The drawing under review shows one solid part. Ordinate dimensions are in mm from its lowest x, y, z. Give positions to 0.01 mm unless a question says otherwise; leave off trailing zeros. Loops run counter-clockwise (first coordinate to the right, second up) from the corner with the lowest first, then second, coordinate; pieces in that order, holes last. Notation, with made-up numbers: (46.5, 87) - (88.5, 87) arc R31 cw to (88.5, 117) - close; hole circle Ø11 at (6, 61). An arc over 180 degrees is marked (long way). One line per item, written item: value. Start each with the question number.
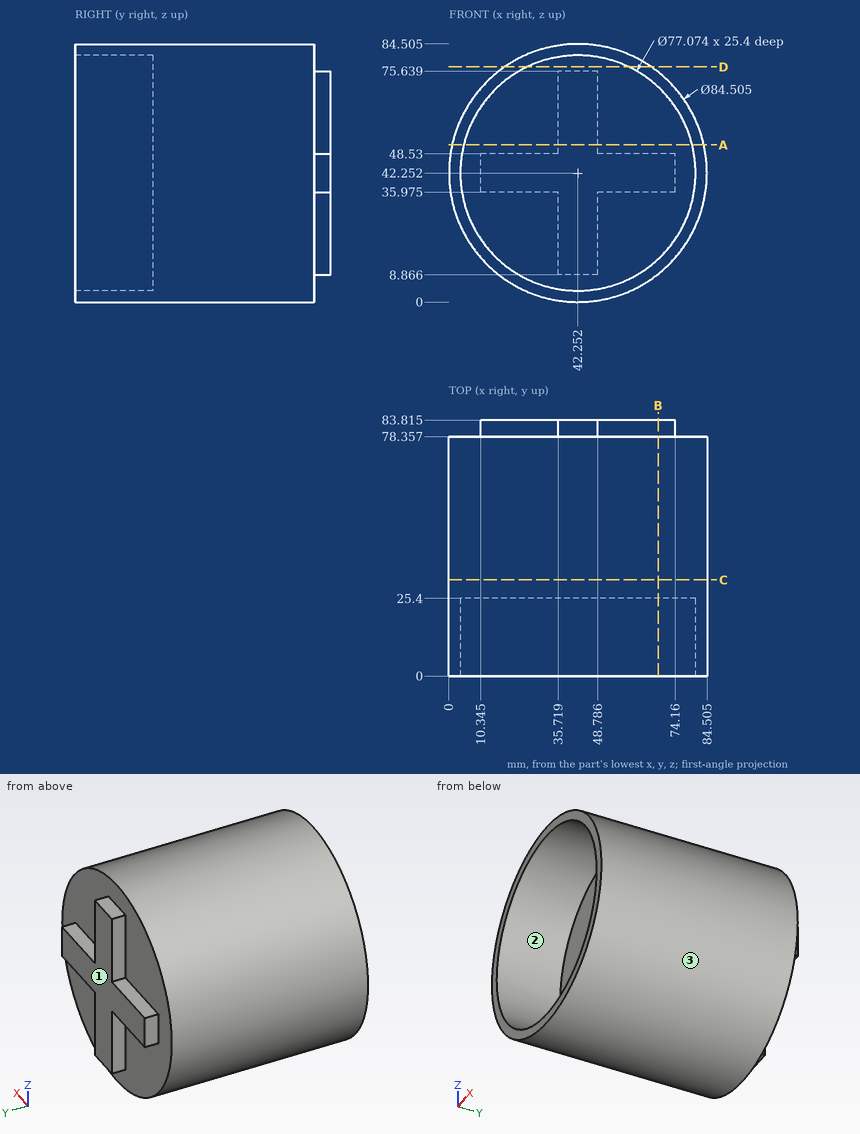
(1) To check wall thickness, follow L1, parallel to Y at x = 25, z = 58; L2, parallel to Y at x = 44, z = 17 (1 decimal); L3, parallel to X at y = 15, z = 13 (1 decimal). State the ranges of each line that lie inside material, in increasing order. Write a range as from..to.
(2) Take a section at B-B on x = 68.5. State the section outline as (y, z) points (1 decimal), and give its area (3 significant figures).
(3) Take a section at D-D on z = 77. State the section outline as (x, y) points, and give its area (3 significant figures).
(4) Take a section at A-A on z = 51.5. State the section outline as (x, y) points (1 decimal).
(5) Take a section at C-C on y = 31.5. State the section outline as (x, z) points (1 decimal), and give its area (3 significant figures).
(6) For pin 1 Ø6 at (y, z) = (68.5, 27) entering from -X (1 decimal); pin 2 Ø10 at (x, y) = (15.5, 51.5) entering from -Z; pin 3 Ø6 at (y, z) = (81, 40) entering from -X, all flat-tipped, find the tip position at first contact; note any pin that passes through.
(7) Draft analysis for pull direction Z (two halves, no side actions). For the marked faces 1, 2 and 3, state which applies: pulls with the +Z half, pulls with the -Z half, needs draft (parallel to the pull), parting line crosses it, or undercut.
Here are the results:
1. L1: 25.4..78.36
1. L2: 25.4..83.8
1. L3: 11.8..17.2, 67.3..72.7
2. outline: (0, 9.1) - (78.4, 9.1) - (78.4, 36) - (83.8, 36) - (83.8, 48.5) - (78.4, 48.5) - (78.4, 75.4) - (0, 75.4) - (0, 70.5) - (25.4, 70.5) - (25.4, 14) - (0, 14) - close
2. area: 3,820 mm²
3. outline: (18.21, 0) - (25.59, 0) - (25.59, 25.4) - (58.92, 25.4) - (58.92, 0) - (66.29, 0) - (66.29, 78.36) - (18.21, 78.36) - close
3. area: 2,920 mm²
4. outline: (1, 0) - (4.8, 0) - (4.8, 25.4) - (79.7, 25.4) - (79.7, 0) - (83.5, 0) - (83.5, 78.4) - (48.8, 78.4) - (48.8, 83.8) - (35.7, 83.8) - (35.7, 78.4) - (1, 78.4) - close
5. outline: circle Ø84.5 at (42.3, 42.3)
5. area: 5,610 mm²
6. pin 1: x = 1.8
6. pin 2: z = 6.03
6. pin 3: x = 0.01
7. face 1: needs draft
7. face 2: undercut
7. face 3: parting line crosses it
